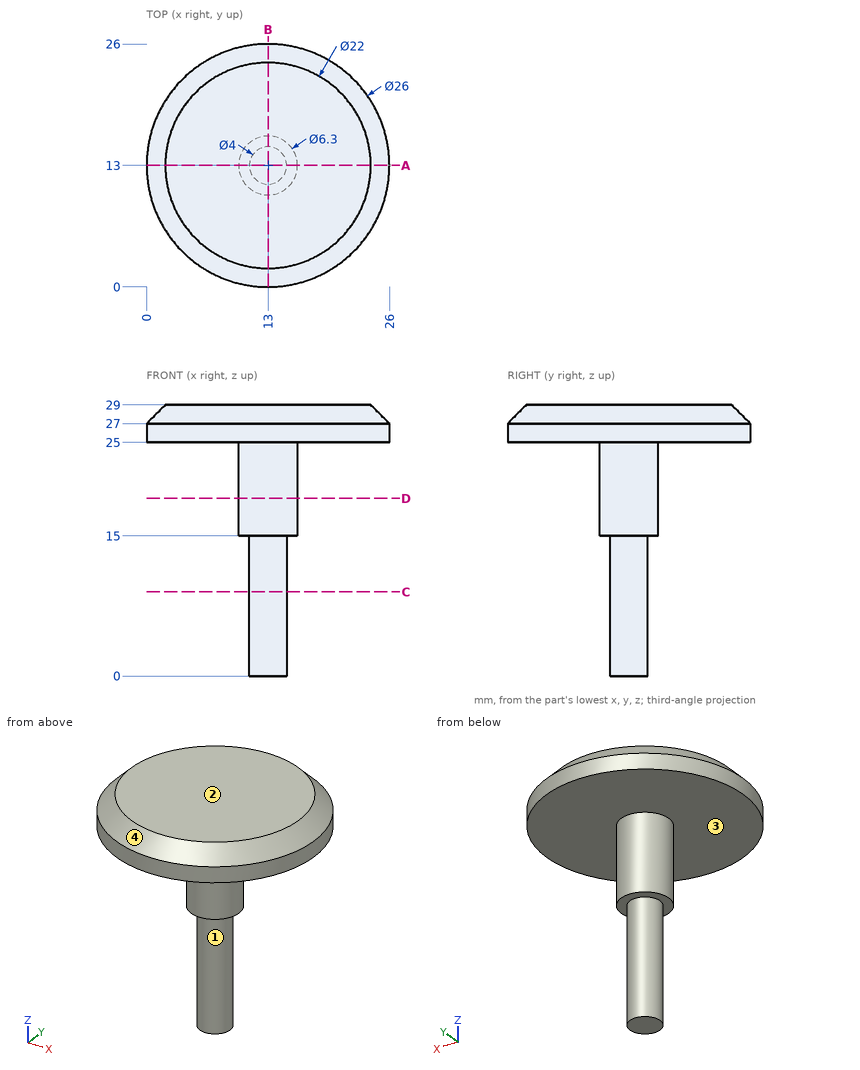
Drawing for the job (mm, zero at the part's lowest x, y, z). A direction names the side the tool comes from. Round coordinates to 2 decimals unless told otherwise and drop trailing zeros. Order: outer loops, then holes, each group sorted by start corner. A loop starts at its lowest first (then second) coordinate and runs counter-clockwise, first axis right, second up.
Item 1: Probe line 1 along Z through (x, y) = (11.25, 19); line 2 along Y through (x, z) = (11.5, 16.5); line 3 along X through (y, z) = (12, 22.75). List the from-to ranges inside material, lowest first.
Item 2: Tool access for the marked faces 1 and 2: list every direction of +Z, -Z, +X, -X, +Y, -Y with a clear straight run to the whole face (end or side of a thin tool).
Item 3: Saw through at D-D on z = 19. Write the cut outline in (x, y).
Item 4: Mould opens along Y. For the marked faces 3 and 4 say: pulls with the +Y half, pulls with the -Y half, needs draft (parallel to the pull), parting line crosses it, or undercut.
Item 5: Saw through at A-A on y = 13. Write the cut outline in (x, z).
Item 6: Saw through at C-C on z = 9. Write the cut outline in (x, y).
Item 7: Pin check, flat tips, straight feed: pin 1 (6 mm diameter, centred on x = 8, y = 18.5, fed in from -Z); pin 2 (3 mm diameter, centred on x = 12.5, z = 9, fed in from +Y). Stop position of each tip, or through.
Reported:
1. line 1: z = 25 to 29
1. line 2: y = 10.23 to 15.77
1. line 3: x = 10.01 to 15.99
2. face 1: -Z
2. face 2: +Z, +X, -X, +Y, -Y
3. outline: circle Ø6.3 at (13, 13)
4. face 3: needs draft
4. face 4: parting line crosses it
5. outline: (0, 25) - (9.85, 25) - (9.85, 15) - (11, 15) - (11, 0) - (15, 0) - (15, 15) - (16.15, 15) - (16.15, 25) - (26, 25) - (26, 27) - (24, 29) - (2, 29) - (0, 27) - close
6. outline: circle Ø4 at (13, 13)
7. pin 1: stops at z = 25
7. pin 2: stops at y = 15
